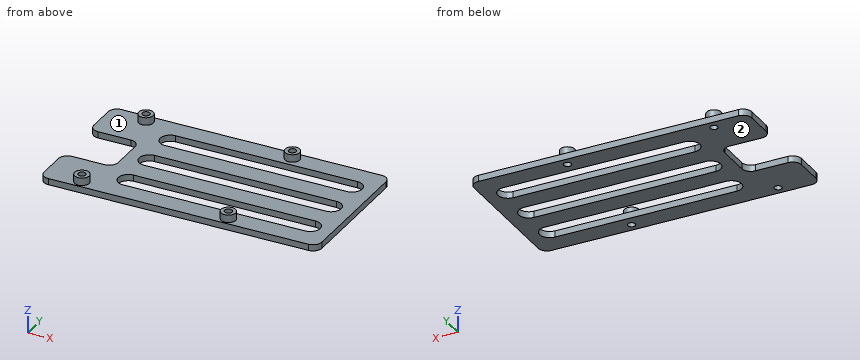
```python
from build123d import *

# Parameters (mm, degrees)
SKETCH_W            = 110
SKETCH_H            = 28
PAD_DEPTH           = 2.5
SKETCH001_R         = 2.9
PAD001_DEPTH        = 3
SKETCH002_R         = 1.5
POCKET_DEPTH        = 5.501
POCKET001_DEPTH     = 2.501
LINEARPATTERN_COUNT = 2
LINEARPATTERN_PITCH = 16
SKETCH004_W         = 20
SKETCH004_H         = 10
POCKET002_DEPTH     = 2.501
FILLET_R            = 3.5


with BuildPart() as part:
    # Sketch → Pad (new body)
    with BuildSketch(Plane.XY):
        with Locations((55, 14)):
            Rectangle(SKETCH_W, SKETCH_H)
    extrude(amount=PAD_DEPTH)

    # Sketch001 (on Face6 of Pad) → Pad001 (join)
    with BuildSketch(Plane.XY.offset(2.5)):
        with Locations((15, 24.5)):
            Circle(SKETCH001_R)
        with Locations((73, 24.5)):
            Circle(SKETCH001_R)
    extrude(amount=PAD001_DEPTH)

    # Sketch002 (on Face9 of Pad001) → Pocket (cut, through all)
    with BuildSketch(Plane.XY.offset(5.5)):
        with Locations((15, 24.5)):
            Circle(SKETCH002_R)
        with Locations((73, 24.5)):
            Circle(SKETCH002_R)
    extrude(amount=-POCKET_DEPTH, mode=Mode.SUBTRACT)

    # Sketch003 (on Face5 of Pocket) → Pocket001 (cut, through all)
    with BuildSketch(Plane.XY.offset(2.5)):
        with BuildLine():
            ThreePointArc((29, 4), (25, 0), (29, -4))
            Line((29, -4), (101, -4))
            ThreePointArc((101, -4), (105, 0), (101, 4))
            Line((29, 4), (101, 4))
        make_face()
    pocket001 = extrude(amount=-POCKET001_DEPTH, mode=Mode.SUBTRACT)

    # LinearPattern: Pocket001 ×2
    with Locations(*[(0, i * LINEARPATTERN_PITCH, 0) for i in range(1, LINEARPATTERN_COUNT)]):
        add(pocket001, mode=Mode.SUBTRACT)

    # Sketch004 (on Face4 of LinearPattern) → Pocket002 (cut, through all)
    with BuildSketch(Plane.XY.offset(2.5)):
        with Locations((10, 5)):
            Rectangle(SKETCH004_W, SKETCH004_H)
    extrude(amount=-POCKET002_DEPTH, mode=Mode.SUBTRACT)

    # Fillet
    fillet_edges = [part.edges().sort_by_distance(p)[0] for p in [
        (20, 10, 1.25),
        (0, 10, 1.25),
        (0, 28, 1.25),
        (110, 28, 1.25),
    ]]
    fillet(fillet_edges, radius=FILLET_R)

    # Mirrored: part across XZ


with BuildPart() as part_1:
    add(part.part)
    add(part.part.mirror(Plane.XZ))


solid = part_1.part
```
Source: CAD feature listing. Evaluate the final solid. Frame: model axes, mm. Face numbers are marked on the shaded views. Give positions to 0.01 mm unless a question says otherwise; leave off trailing zeros. Write each loop counter-clockwise with the first axis right and the second up, starting at its lowest first coordinate (ties: lowest second). Pieces come first, ordered by that corner, then holes.
1. First-contact query: pin 1 (3 mm diameter, centred on y = 0.5, z = 0.5, fed in from -X). Flat tip, straight axial feed; report the tip coordinate or a pass-through.
2. Section query A-A (x = 73). Count the separate pieces of the cut face and the enclosed holes in it, then the cut area to 3 significant figures.
3. Pull-direction query (X, two-part tool) for the marked faces 1 and 2; classes: +X half, -X half, draft (parallel to the pull), parting line (faces both ways), or undercut.
4. Section query D-D (x = 47.5). Return the cut outline in (y, z).
5. Section query B-B (z = 4.25). Return the cut outline in (x, y), then the cut area to 3 significant figures.
6. Material intervals for line 1 along Y through (x, z) = (15, 1.35); line 2 along Y through (x, z) = (73, 1.5); line 3 along Y through (x, z) = (15, 2.8), sorted ascending.
7. Section query C-C (y = -16). Return the cut outline in (x, z), then the cut area to 3 significant figures.
Output values:
1. pin 1: stops at x = 20
2. separate pieces: 6
2. enclosed holes: 0
2. area: 81.8 mm2
3. face 1: undercut
3. face 2: draft
4. outline: (-28, 0) - (-20, 0) - (-20, 2.5) - (-28, 2.5) - close; (-12, 0) - (-4, 0) - (-4, 2.5) - (-12, 2.5) - close; (4, 0) - (12, 0) - (12, 2.5) - (4, 2.5) - close; (20, 0) - (28, 0) - (28, 2.5) - (20, 2.5) - close
5. outline: circle Ø5.8 at (15, -24.5); circle Ø5.8 at (15, 24.5); circle Ø5.8 at (73, -24.5); circle Ø5.8 at (73, 24.5); hole circle Ø3 at (15, -24.5); hole circle Ø3 at (15, 24.5); hole circle Ø3 at (73, -24.5); hole circle Ø3 at (73, 24.5)
5. area: 77.4 mm2
6. line 1: y = -28 to -26, -23 to -10, 10 to 23, 26 to 28
6. line 2: y = -28 to -26, -23 to -20, -12 to -4, 4 to 12, 20 to 23, 26 to 28
6. line 3: y = -27.4 to -26, -23 to -21.6, 21.6 to 23, 26 to 27.4
7. outline: (0, 0) - (25, 0) - (25, 2.5) - (0, 2.5) - close; (105, 0) - (110, 0) - (110, 2.5) - (105, 2.5) - close
7. area: 75.0 mm2
